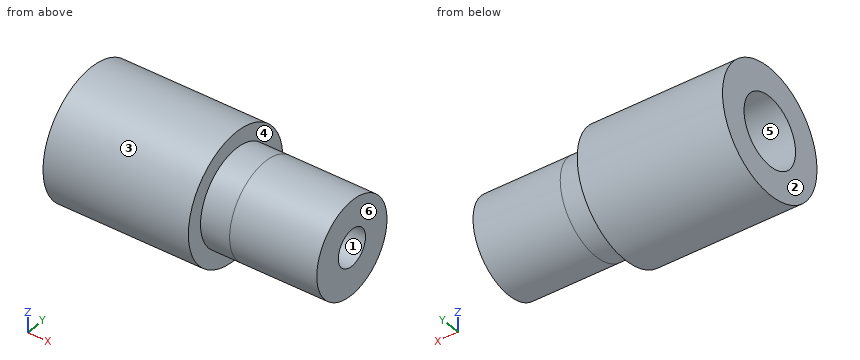
Autodesk Fusion 360 part; units mm, degrees
sketch "Boceto1" plane through (0, 0, 0) normal (1, 0, 0) x (0, 1, 0)
  circle A0 centre (4.4228, -4.6349) radius 3.175
  circle A1 centre (4.4228, -4.6349) radius 8.175
  dimension "d1" = 6.35
  dimension "d2" = 5
extrude "Extruir1" add sketch "Boceto1" along normal blind 15
sketch "Boceto2" plane through (0, 0, 0) normal (-1, 0, 0) x (0, -1, 0)
  circle A0 centre (-4.4228, -4.6349) radius 3.175
  circle A1 centre (-4.4228, -4.6349) radius 8.175
  circle A2 centre (-4.4228, -4.6349) radius 8.175
extrude "Extruir2" add sketch "Boceto2" along normal blind 5 contours A0 | A1 A2
sketch "Boceto3" plane through (-5, 0, 0) normal (-1, 0, 0) x (0, -1, 0)
  circle A0 centre (-4.4228, -4.6349) radius 8.175
  circle A1 centre (-4.4228, -4.6349) radius 11
  dimension "d7" = 22
extrude "Extruir3" add sketch "Boceto3" along normal blind 25 contours A0 | A1
sketch "Boceto4" plane through (-30, 0, 0) normal (-1, 0, 0) x (0, -1, 0)
  circle A0 centre (-4.4228, -4.6349) radius 11
  circle A1 centre (-4.4228, -4.6349) radius 6
  dimension "d10" = 12
extrude "Extruir4" cut sketch "Boceto4" against normal blind 23 contours A1
CAD build for the part. Positions are in the model's coordinates, mm. Face numbers are marked on the shaded views. A direction names the side the tool comes from. Round coordinates to 2 decimals unless told otherwise and drop trailing zeros. Loops run counter-clockwise (first coordinate to the right, second up) from the corner with the lowest first, then second, coordinate; pieces in that order, holes last.
(1) Drop flat-ended pins along their axis: pin 1 (1.5 mm diameter, centred on x = -4.5, z = -7.5, fed in from +Y); pin 2 (5.5 mm diameter, centred on y = 4.42, z = -4.63, fed in from -X); pin 3 (12 mm diameter, centred on x = 9, z = -9.5, fed in from +Y). Give the stop position or say it passes through.
(2) Cut at C-C (x = -4.5). Give the cut face in (y, z) (3 decimals), plus the area to 3 significant figures.
(3) Wall check: line 1 along X through (y, z) = (-0.25, -11.5); line 2 along Z through (x, y) = (-24, 0.75); line 3 along Y through (x, z) = (-7.5, -1.5). Give the ranges that are in metal, low to high.
(4) Cut at D-D (x = 10). Give the cut face in (y, z) (3 decimals).
(5) Two-plate mould, pull along Y, no slides. Class the marked faces 1, 2 and 3: +Y half, -Y half, draft (parallel to the pull), parting line (faces both ways), or undercut.
(6) Cut at B-B (y = 11). Give the cut face in (x, z), plus the area to 3 significant figures.
(7) Cut at A-A (z = -2.75). Give the cut face in (x, y).
(8) Which spindle directions (+Z, -Z, +X, -X, +Y, -Y) get a long thin tool onto all of the face, cutting with end or side? Do the marked faces 4, 5 and 6. Say none if no direction does.
Findings below:
1. pin 1: stops at y = 15.18
1. pin 2: stops at x = -7
1. pin 3: stops at y = 12.6
2. outline: circle Ø16.35 at (4.423, -4.635)
2. area: 210 mm2
3. line 1: x = -30 to -5
3. line 2: z = -15 to -9.38, 0.11 to 5.73
3. line 3: y = -6.12 to -0.69, 9.54 to 14.97
4. outline: circle Ø16.35 at (4.423, -4.635); hole circle Ø6.35 at (4.423, -4.635)
5. face 1: undercut
5. face 2: draft
5. face 3: parting line
6. outline: (-30, -13.45) - (-5, -13.45) - (-5, -9.49) - (15, -9.49) - (15, 0.22) - (-5, 0.22) - (-5, 4.18) - (-30, 4.18) - close
6. area: 635 mm2
7. outline: (-30, -6.41) - (-5, -6.41) - (-5, -3.53) - (15, -3.53) - (15, 1.87) - (0, 1.87) - (0, 6.98) - (15, 6.98) - (15, 12.38) - (-5, 12.38) - (-5, 15.26) - (-30, 15.26) - (-30, 10.12) - (-7, 10.12) - (-7, -1.27) - (-30, -1.27) - close
8. face 4: +X
8. face 5: -X
8. face 6: +Z, -Z, +X, +Y, -Y
